Read the model definition and answer for the solid it produces. Units are mm, in the model's axes. A direction names the side the tool comes from. Round coordinates to 2 decimals unless told otherwise and drop trailing zeros. Write each loop counter-clockwise with the first axis right and the second up, starting at its lowest first coordinate (ties: lowest second). Pieces come first, ordered by that corner, then holes. Notation, with made-up numbers: (-5, -17) - (10, -17) arc R29 cw to (10, 10) - close; hole circle Ø4 at (39.5, 24.25). An arc over 180 degrees is marked (long way). Use one line per item in the form item = value. Start each with the question number.
1) For a pull along Z with two mould halves and no side action, classify faces 4 (the face through (0, 0, -59.5)), 5 (the face through (0, 0, -30)), 6 (the face through (1.172, 8.923, -54.43)), 7 (the face through (-14.985, 0.66, -32.528)) as released by +Z, released by -Z, zero draft, split by the parting line, or undercut.
2) The part is cut by section B-B, the plane z = -14. Give the vertices of the cut face in (x, y).
3) The part is cut by section D-D, the plane z = -70. Give the vertices of the cut face in (x, y).
4) Each of these flat-tipped pins is pushed along its axis until it touches: pin 1 (9.5 mm diameter, centred on x = 1, y = 4, fed in from +Z); pin 2 (4 mm diameter, centred on y = 14, z = -31, fed in from +X); pin 3 (12 mm diameter, centred on y = -2.5, z = -61, fed in from +X); pin 4 (6.5 mm diameter, centred on x = 0, y = 0, fed in from -Z). Where does it stop, or does it pass through?
5) Consider line 1 along Y through (x, z) = (0, -15.5); line 2 along Y through (x, z) = (0, -71.5); line 3 along Z through (x, y) = (-1, 2). Determine where each line is inside the solid, lowest interval first. Write a range as from..to.
6) For faces 1 (the face through (20.03, 6.31, -12.37)), 2 (the face through (0.867, -3.905, -90.427)), 3 (the face through (-3, 0, -15)), determine the directions among +Z, -Z, +X, -X, +Y, -Y from which every point of the face is accessible in a straight line to the end or side of a thin tool.
7) The part is cut by section C-C, the plane z = -39. Give the vertices of the cut face in (x, y).
from build123d import *

# Parameters (mm, degrees)
SKETCH2_R           = 9
BOSS_EXTRUDE1_DEPTH = 10
SKETCH3_R           = 9
BOSS_EXTRUDE2_DEPTH = 61
BOSS_EXTRUDE2_TAPER = 3
SKETCH4_R           = 4
CUT_EXTRUDE1_DEPTH  = 61


with BuildPart() as part:
    # Sketch1 → Revolve1 (revolve)
    with BuildSketch(Plane(origin=(0, 0, 0), x_dir=(1, 0, 0), z_dir=(0, 1, 0))):
        Polygon((3, 0), (15, 0), (21, 4), (21, 20.5), (16, 20.5), (16, 30.5), (15, 30.5), (15, 34.5), (16, 34.5), (16, 49.5), (0, 49.5), (0, 30), (3, 30), align=None)
    revolve(axis=Axis((0, 0, -75.9090067), (0, 0, 1)))

    # Sketch2 → Boss-Extrude1 (add)
    with BuildSketch(Plane(origin=(0, 0, -49.5), x_dir=(-1, 0, 0), z_dir=(0, 0, -1))):
        Circle(SKETCH2_R)
    extrude(amount=BOSS_EXTRUDE1_DEPTH)

    # Sketch3 → Boss-Extrude2 (add)
    with BuildSketch(Plane(origin=(0, 0, -59.5), x_dir=(-1, 0, 0), z_dir=(0, 0, -1))):
        Circle(SKETCH3_R)
    extrude(amount=BOSS_EXTRUDE2_DEPTH, taper=BOSS_EXTRUDE2_TAPER)

    # Sketch4 → Cut-Extrude1 (cut)
    with BuildSketch(Plane(origin=(0, 0, -120.5), x_dir=(-1, 0, 0), z_dir=(0, 0, -1))):
        Circle(SKETCH4_R)
    extrude(amount=-CUT_EXTRUDE1_DEPTH, mode=Mode.SUBTRACT)


solid = part.part
Geometry results:
q1.face_4 = released by -Z
q1.face_5 = released by +Z
q1.face_6 = zero draft
q1.face_7 = undercut
q2.outline = circle Ø42 at (0, 0); hole circle Ø6 at (0, 0)
q3.outline = circle Ø16.9 at (0, 0); hole circle Ø8 at (0, 0)
q4.pin_1 = 0
q4.pin_2 = 10.51
q4.pin_3 = 9
q4.pin_4 = -59.5
q5.line_1 = -21..-3, 3..21
q5.line_2 = -8.37..-4, 4..8.37
q5.line_3 = -59.5..-30
q6.face_1 = +Z, -Z
q6.face_2 = -Z
q6.face_3 = +Z
q7.outline = circle Ø32 at (0, 0)
